Solid Edge part; units mm, degrees
sketch "Sketch1" plane through (0, 0, 0) normal (0, 0, 1) x (1, 0, 0)
  circle A0 centre (0, 0) radius 22.86
extrude "Protrusion1" add sketch "Sketch1" along normal blind 12.7
sketch "Sketch2" plane through (0, 0, 0) normal (0, 0, 1) x (1, 0, 0)
  circle A0 centre (0, 0) radius 2.54
extrude "ExtrudedCutout_2" cut sketch "Sketch2" along normal blind 15.2909
sketch "Sketch3" plane through (0, 0, 0) normal (0, 0, 1) x (1, 0, 0)
  line L0 (0, 20.32) -> (-2.54, 20.32)
  line L1 (-2.54, 20.32) -> (-3.8208, 22.5384)
  line L2 (2.54, 20.32) -> (3.8208, 22.5384)
  line L3 (0, 20.32) -> (2.54, 20.32)
  arc A0 (-3.8208, 22.5384) -> (3.8208, 22.5384) centre (0, 0) cw
extrude "Cutout1" cut sketch "Sketch3" along normal up to vertex (12.7 mm away)
pattern_circular "Pattern1" count 10 over 360 about axis through (0, 0, 12.7) along (0, 0, 1) of "Cutout1"
sketch "Sketch4" plane through (0, 0, 12.7) normal (0, 0, 1) x (0.5, 0.866, 0)
  circle A0 centre (0, 0) radius 6.35
extrude "ExtrudedProtrusion_3" add sketch "Sketch4" along normal blind 2.54
Here's how the part is built. I have some questions about the finished solid (model axes, mm). A direction names the side the tool comes from. Coordinates: 2 decimals unless noted, no trailing zeros. Order: outer loops, then holes, each group sorted by start corner. A loop starts at its lowest first (then second) coordinate and runs counter-clockwise, first axis right, second up.
1) I need wall thicknesses on line 1 (X direction, y = 0, z = 7.5); line 2 (Y direction, x = 0, z = 5.25); line 3 (Z direction, x = -15.5, y = 0). Which ranges of each line are inside material? Lowest first, please.
2) Imagine slicing it at B-B on x = 0. List the corners of the cut face in (y, z) for me, and give its area (3 significant figures).
3) Imagine slicing it at C-C on x = 5.5. List the corners of the cut face in (y, z) for me, and give its area (3 significant figures).
4) Which directions (+Z, -Z, +X, -X, +Y, -Y) give clear straight access to the entire face, cutting with the end or side of a thin tool? Please do faces 4 (the face through (-7.109, 21.727, 6.261)), 5 (the face through (10, 19, 6)), 6 (the face through (0, 0, 15.24)), 7 (the face through (-19.336, -6.245, 6.261)), 8 (the face through (0, -20.32, 6)).
5) We'd pull the mould along Y, two halves only. Please class faces 1 (the face through (-19.314, 6.313, 6.261)), 2 (the face through (-7.02, -21.756, 6.261)), 3 (the face through (-15.15, 15.46, 6.26)): +Y half, -Y half, draft (parallel to the pull), parting line (faces both ways), or undercut.
6) Imagine slicing it at D-D on y = -19. List the corners of the cut face in (x, z) for me.
7) Imagine slicing it at A-A on y = 0. List the corners of the cut face in (x, z) for me.
8) Will these pins go through, and if not, where does the flat tip stop? pin 1 (5 mm diameter, centred on x = 6.5, z = 7.5, fed in from +Y); pin 2 (6 mm diameter, centred on x = -7.5, z = 5.5, fed in from -Y); pin 3 (3 mm diameter, centred on y = 3.5, z = 8, fed in from -X).
Response values:
1. line 1: x = -22.86 to -2.54, 2.54 to 22.86
1. line 2: y = -20.32 to -2.54, 2.54 to 20.32
1. line 3: z = 0 to 12.7
2. outline: (-20.32, 0) - (-2.54, 0) - (-2.54, 12.7) - (2.54, 12.7) - (2.54, 0) - (20.32, 0) - (20.32, 12.7) - (6.35, 12.7) - (6.35, 15.24) - (-6.35, 15.24) - (-6.35, 12.7) - (-20.32, 12.7) - close
2. area: 484 mm2
3. outline: (-22.19, 0) - (22.19, 0) - (22.19, 12.7) - (3.17, 12.7) - (3.17, 15.24) - (-3.17, 15.24) - (-3.17, 12.7) - (-22.19, 12.7) - close
3. area: 580 mm2
4. face 4: +Z, -Z, -X, +Y
4. face 5: +Z, -Z, +X
4. face 6: +Z, +X, -X, +Y, -Y
4. face 7: +Z, -Z, -X
4. face 8: +Z, -Z, -Y
5. face 1: undercut
5. face 2: -Y half
5. face 3: +Y half
6. outline: (-10, 0) - (10, 0) - (10, 12.7) - (-10, 12.7) - close
7. outline: (-22.86, 0) - (-2.54, 0) - (-2.54, 12.7) - (2.54, 12.7) - (2.54, 0) - (22.86, 0) - (22.86, 12.7) - (6.35, 12.7) - (6.35, 15.24) - (-6.35, 15.24) - (-6.35, 12.7) - (-22.86, 12.7) - close
8. pin 1: stops at y = 22.51
8. pin 2: stops at y = -22.41
8. pin 3: stops at x = -22.77
